Can you work these out from the model? Positions are in its coordinate system, mm. A direction names the side the tool comes from. Round coordinates to 2 decimals unless told otherwise and drop trailing zeros. Loops run counter-clockwise (first coordinate to the right, second up) from the corner with the lowest first, then second, coordinate; pieces in that order, holes last. Notation, with made-up numbers: M -3.5,65.5 L 0.5,65.5 A17 ccw 0.5,97.5 Z; hole C 65.5,16.5 d10. An arc over 180 degrees is marked long. Return JSON: item names as keys, results as strings.
```python
from build123d import *

# Parameters (mm, degrees)
SKETCH2_W                     = 8
SKETCH2_H                     = 10.25
CUT_FLATS_TOP_BOT_LEFT_DEPTH  = 30
SKETCH3_W                     = 8
SKETCH3_H                     = 10.25
CUT_FLATS_SIDES_LEFT_DEPTH    = 30
SKETCH4_W                     = 8
SKETCH4_H                     = 10.25
CUT_FLATS_TOP_BOT_RIGHT_DEPTH = 30
SKETCH5_W                     = 8
SKETCH5_H                     = 10.25
CUT_FLATS_SIDES_RIGHT_DEPTH   = 30


with BuildPart() as part:
    # Sketch1 → Revolve-Shaft (revolve)
    with BuildSketch(Plane.XY, mode=Mode.PRIVATE) as revolve_shaft_sk:
        Polygon((0, 0), (0, 5), (16, 5), (16, 6), (26, 6), (26, 7.5), (41, 7.5), (41, 9), (43, 7.5), (43, 6), (59, 6), (59, 0), align=None)
    revolve(revolve_shaft_sk.sketch.rotate(Axis((0, 0, 0), (1, 0, 0)), 90), axis=Axis((0, 0, 0), (1, 0, 0)))

    # Sketch2 → Cut-Flats Top-Bot Left (cut)
    with BuildSketch(Plane(origin=(0, 0, 0), x_dir=(1, 0, 0), z_dir=(0, 1, 0))):
        with Locations((8, 9.875)):
            Rectangle(SKETCH2_W, SKETCH2_H)
        with Locations((8, -9.875)):
            Rectangle(SKETCH2_W, SKETCH2_H)
    extrude(amount=-CUT_FLATS_TOP_BOT_LEFT_DEPTH, mode=Mode.SUBTRACT)

    # Sketch3 → Cut-Flats Sides Left (cut)
    with BuildSketch(Plane.XY):
        with Locations((8, 9.875)):
            Rectangle(SKETCH3_W, SKETCH3_H)
        with Locations((8, -9.875)):
            Rectangle(SKETCH3_W, SKETCH3_H)
    extrude(amount=-CUT_FLATS_SIDES_LEFT_DEPTH, mode=Mode.SUBTRACT)

    # Sketch4 → Cut-Flats Top-Bot Right (cut)
    with BuildSketch(Plane(origin=(0, 0, 0), x_dir=(1, 0, 0), z_dir=(0, 1, 0))):
        with Locations((51, 9.875)):
            Rectangle(SKETCH4_W, SKETCH4_H)
        with Locations((51, -9.875)):
            Rectangle(SKETCH4_W, SKETCH4_H)
    extrude(amount=-CUT_FLATS_TOP_BOT_RIGHT_DEPTH, mode=Mode.SUBTRACT)

    # Sketch5 → Cut-Flats Sides Right (cut)
    with BuildSketch(Plane.XY):
        with Locations((51, 9.875)):
            Rectangle(SKETCH5_W, SKETCH5_H)
        with Locations((51, -9.875)):
            Rectangle(SKETCH5_W, SKETCH5_H)
    extrude(amount=-CUT_FLATS_SIDES_RIGHT_DEPTH, mode=Mode.SUBTRACT)


solid = part.part
```
Q1. Suppose I cut it at B-B, the plane x = 14.5. Please give me the cut outline in (y, z).
Results:
{"outline": "C 0,0 d10"}
Q2. If I drill on line 1 along X through (y, z) = (5.75, -1.5); line 2 along X through (y, z) = (-1, -7); line 3 along X through (y, z) = (-5.25, 1.25), over which ranges is the centre line in solid material (lowest first)?
Results:
{"line 1": "x = 16 to 47, 55 to 59", "line 2": "x = 26 to 43", "line 3": "x = 16 to 59"}
Q3. On a 3-axis mill with a long thin cutter (end or side, diameter ignored), from which of +Z, -Z, +X, -X, +Y, -Y can I reach the whole of each face in a straight line? I mean faces 1 (the flat face through (43, -6, 2)), 2 (the flat face through (41, -7.4, 2)), 3 (the flat face through (51, 0, -5)), 4 (the flat face through (47, 5, -1)), 5 (the flat face through (8, -1, 4.75)). Say none if no direction works.
Results:
{"face 1": "+X", "face 2": "-X", "face 3": "-Z, -Y", "face 4": "-Z, +Y", "face 5": "+Z, -Y"}
Q4. Thinking about a two-plate mould opening in X: for faces 6 (the cylindrical face through (21.07, -1.802, 5.723)), 7 (the flat face through (16, -4, 4)), 8 (the flat face through (55, -5, -1)), which applies, pulls with the +X half, pulls with the -X half, needs draft (parallel to the pull), parting line crosses it, or undercut?
Results:
{"face 6": "needs draft", "face 7": "pulls with the -X half", "face 8": "undercut"}
Q5. Suppose I cut it at A-A, the plane x = 48.5. Please give me the cut outline in (y, z).
Results:
{"outline": "M -6,0 L -4.75,0 L -4.75,-3.67 A6 ccw -3.67,-4.75 L 0,-4.75 L 0,-6 A6 ccw 4.75,-3.67 L 4.75,0 L 6,0 A6 ccw 0,6 L 0,4.75 L -3.67,4.75 A6 ccw Z"}
Q6. I'm going to push flat-ended pins straight in: pin 1 Ø1.5 at (x, y) = (31.5, -6.5) entering from -Z; pin 2 Ø1 at (x, z) = (9.5, -3.5) entering from -Y; pin 3 Ø3 at (x, y) = (6, -1) entering from +Z. Where does each tip first touch, or does it pass through?
Results:
{"pin 1": "stops at z = -4.82", "pin 2": "stops at y = -4", "pin 3": "stops at z = 5"}
